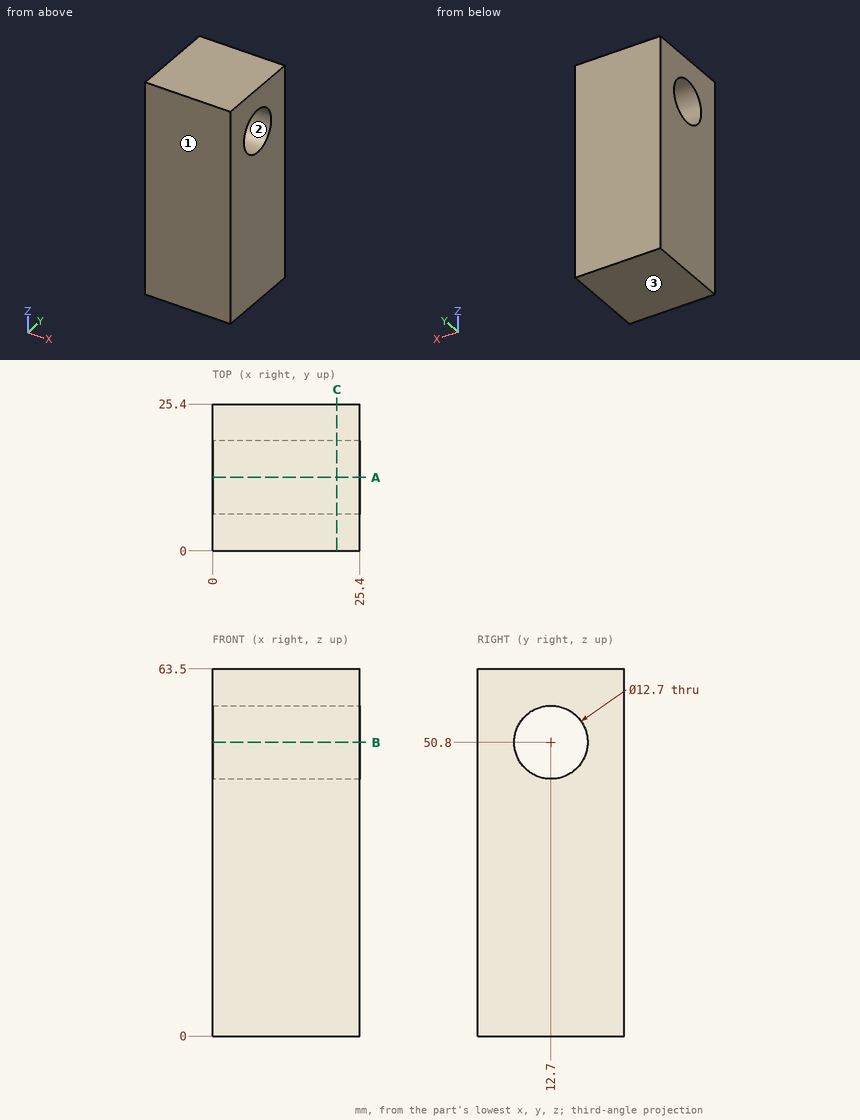
Print and shaded views of the part. All mm, measured from the part's lowest x, y and z. Coordinates: 2 decimals unless noted, no trailing zeros. Write each loop counter-clockwise with the first axis right and the second up, starting at its lowest first coordinate (ties: lowest second). Pieces come first, ordered by that corner, then holes.
(1) Cut at B-B, the plane z = 50.8. List the corners of the cut face in (x, y).
(2) Drill centre lines: probe 1 along Y at (x, z) = (20.25, 50.8); probe 2 along Z at (x, y) = (14.5, 16.25); probe 3 along Z at (x, y) = (18.5, 7.75). Where is each one in solid material? Low to high.
(3) Cut at A-A, the plane y = 12.7. List the corners of the cut face in (x, z).
(4) Cut at C-C, the plane x = 21.5. List the corners of the cut face in (y, z), and give its area (3 significant figures).
(5) Two-plate mould, pull along Z, no slides. Class the marked faces 1, 2 and 3: +Z half, -Z half, draft (parallel to the pull), parting line (faces both ways), or undercut.
Geometry says:
1. outline: (0, 0) - (25.4, 0) - (25.4, 6.35) - (0, 6.35) - close; (0, 19.05) - (25.4, 19.05) - (25.4, 25.4) - (0, 25.4) - close
2. probe 1: y = 0 to 6.35, 19.05 to 25.4
2. probe 2: z = 0 to 45.54, 56.06 to 63.5
2. probe 3: z = 0 to 46.82, 54.78 to 63.5
3. outline: (0, 0) - (25.4, 0) - (25.4, 44.45) - (0, 44.45) - close; (0, 57.15) - (25.4, 57.15) - (25.4, 63.5) - (0, 63.5) - close
4. outline: (0, 0) - (25.4, 0) - (25.4, 63.5) - (0, 63.5) - close; hole circle Ø12.7 at (12.7, 50.8)
4. area: 1,490 mm2
5. face 1: draft
5. face 2: undercut
5. face 3: -Z half
